```python
from build123d import *

# Parameters (mm, degrees)
SKETCH1_R           = 3
SKETCH1_R_2         = 5
SKETCH1_R_3         = 1.25
BOSS_EXTRUDE1_DEPTH = 3
SKETCH2_R           = 1.75
BOSS_EXTRUDE2_DEPTH = 3
BOSS_EXTRUDE3_DEPTH = 30.5


with BuildPart() as part:
    # Sketch1 → Boss-Extrude1 (new body)
    with BuildSketch(Plane.XY):
        with BuildLine():
            Line((-4.824371659, -30.813559322), (-12.302147731, -3.349576271))
            ThreePointArc((-12.302147731, -3.349576271), (0, 12.75), (12.302147731, -3.349576271))
            Line((12.302147731, -3.349576271), (4.824371659, -30.813559322))
            ThreePointArc((4.824371659, -30.813559322), (0, -34.5), (-4.824371659, -30.813559322))
        make_face()
        with Locations((0, -29.5)):
            Circle(SKETCH1_R, mode=Mode.SUBTRACT)
        with Locations((0, -3)):
            Circle(SKETCH1_R_2, mode=Mode.SUBTRACT)
        with Locations((-9.5, 0)):
            Circle(SKETCH1_R_3, mode=Mode.SUBTRACT)
        with Locations((9.5, 0)):
            Circle(SKETCH1_R_3, mode=Mode.SUBTRACT)
    boss_extrude1 = extrude(amount=BOSS_EXTRUDE1_DEPTH)

    # Sketch2 → Boss-Extrude2 (add)
    with BuildSketch(Plane.XY):
        with BuildLine():
            Line((-2.214014265, 12.556298851), (19.806700742, 16.439145041))
            ThreePointArc((19.806700742, 16.439145041), (23.131694024, 14.858482542), (22.729129297, 11.198972206))
            Line((22.729129297, 11.198972206), (12.75, 0))
            ThreePointArc((12.75, 0), (8.195542024, 9.76706665), (-2.214014265, 12.556298851))
        make_face()
        with Locations((20.358155694, 13.311688597)):
            Circle(SKETCH2_R, mode=Mode.SUBTRACT)
    boss_extrude2 = extrude(amount=BOSS_EXTRUDE2_DEPTH)

    # Sketch4 → Boss-Extrude3 (add)
    with BuildSketch(Plane.XY):
        with BuildLine():
            Line((-12.302147731, -3.349576271), (-14.929266375, 6.299167048))
            ThreePointArc((-14.929266375, 6.299167048), (-14.445067335, 10.095245581), (-11.418454038, 12.437098029))
            Line((-11.418454038, 12.437098029), (-4.181896549, 14.407437012))
            Line((-4.181896549, 14.407437012), (2.785985735, 13.437933754))
            Line((2.785985735, 13.437933754), (-2.214014265, 12.556298851))
            ThreePointArc((-2.214014265, 12.556298851), (-10.767030957, 6.828875777), (-12.302147731, -3.349576271))
        make_face()
    boss_extrude3 = extrude(amount=BOSS_EXTRUDE3_DEPTH)

    # Mirror2: Boss-Extrude1, Boss-Extrude2, Boss-Extrude3 across plane
    add(boss_extrude1.mirror(Plane.XY.offset(30.5)))
    add(boss_extrude2.mirror(Plane.XY.offset(30.5)))
    add(boss_extrude3.mirror(Plane.XY.offset(30.5)))


solid = part.part
```
The listing builds one solid part. Answer for the finished solid, in the listing's coordinates (mm). A direction names the side the tool comes from. Give positions to 0.01 mm unless a question says otherwise; leave off trailing zeros. Order: outer loops, then holes, each group sorted by start corner. A loop starts at its lowest first (then second) coordinate and runs counter-clockwise, first axis right, second up. Notation, with made-up numbers: (24.25, 16.5) - (68.25, 16.5) arc R23 ccw to (68.25, 49.5) - close; hole circle Ø5 at (75.25, 64.5). An arc over 180 degrees is marked (long way). Use one line per item in the form item = value. Start each with the question number.
(1) A cutting plane is placed at A-A, the plane x = -9.5. Write down the section's boundary in (y, z).
(2) Flat-ended cylindrical pins translate along their axes: pin 1 Ø5 at (y, z) = (5.5, 31.5) entering from +X; pin 2 Ø6 at (x, y) = (0, -3) entering from +Z. Find the tip coordinate at first contact, or state that the pin passes through.
(3) A cutting plane is placed at C-C, the plane x = 0. Write down the section's boundary in (y, z).
(4) A cutting plane is placed at B-B, the plane y = -16. Write down the section's boundary in (x, z), then the cut area to 3 significant figures.
(5) For faces 1 (the flat face through (0, -9, 61)), 2 (the flat face through (11.18, 14.92, 59.52)), determine the directions among +Z, -Z, +X, -X, +Y, -Y from which every point of the face is accessible in a straight line to the end or side of a thin tool.
(6) A cutting plane is placed at D-D, the plane y = -29.5. Write down the section's boundary in (x, z), then the cut area to 3 significant figures.
(7) The mould has two halves that part along Y. Classify faces 3 (the cylindrical face through (23.105, 14.906, 1.479)), 4 (the cylindrical face through (0.1, -34.5, 1.5)), 5 (the cylindrical face through (8.25, 0.05, 1.48)), 6 (the cylindrical face through (-1.08, -7.88, 1.48)): released by +Y, released by -Y, zero draft, split by the parting line, or undercut.
(8) Consider line 1 (Z direction, x = 7, y = -21); line 2 (Y direction, x = 0, z = 59.8); line 3 (Y direction, x = 0, z = 3.5). Determine where each line is inside the solid, lowest interval first. Write a range as from..to.
Ans:
q1.outline = (-13.64, 0) - (-1.25, 0) - (-1.25, 3) - (-13.64, 3) - close; (-13.64, 58) - (-1.25, 58) - (-1.25, 61) - (-13.64, 61) - close; (1.25, 0) - (12.96, 0) - (12.96, 61) - (1.25, 61) - (1.25, 58) - (8.5, 58) - (8.5, 3) - (1.25, 3) - close
q2.pin_1 = -9.93
q2.pin_2 = through
q3.outline = (-34.5, 0) - (-32.5, 0) - (-32.5, 3) - (-34.5, 3) - close; (-34.5, 58) - (-32.5, 58) - (-32.5, 61) - (-34.5, 61) - close; (-26.5, 0) - (-8, 0) - (-8, 3) - (-26.5, 3) - close; (-26.5, 58) - (-8, 58) - (-8, 61) - (-26.5, 61) - close; (2, 0) - (13.83, 0) - (13.83, 61) - (2, 61) - (2, 58) - (12.95, 58) - (12.95, 3) - (2, 3) - close
q4.outline = (-8.86, 0) - (8.86, 0) - (8.86, 3) - (-8.86, 3) - close; (-8.86, 58) - (8.86, 58) - (8.86, 61) - (-8.86, 61) - close
q4.area = 106 mm^2
q5.face_1 = +Z, +X, -X, +Y, -Y
q5.face_2 = +Z, -Z, +Y
q6.outline = (-5.18, 0) - (-3, 0) - (-3, 3) - (-5.18, 3) - close; (-5.18, 58) - (-3, 58) - (-3, 61) - (-5.18, 61) - close; (3, 0) - (5.18, 0) - (5.18, 3) - (3, 3) - close; (3, 58) - (5.18, 58) - (5.18, 61) - (3, 61) - close
q6.area = 26.2 mm^2
q7.face_3 = split by the parting line
q7.face_4 = released by -Y
q7.face_5 = undercut
q7.face_6 = undercut
q8.line_1 = 0..3, 58..61
q8.line_2 = -34.5..-32.5, -26.5..-8, 2..13.83
q8.line_3 = 12.95..13.83
